Part model, mm, in its own coordinate system. Give positions to 0.01 mm unless a question says otherwise; leave off trailing zeros. Loops run counter-clockwise (first coordinate to the right, second up) from the corner with the lowest first, then second, coordinate; pieces in that order, holes last. Notation, with made-up numbers: M -3,-17 L 12,-17 A8 cw 12,-7 Z; hole C 21,46.5 d2. An arc over 180 degrees is marked long. Put each result on its own line as item: value. Start each with the question number.
Autodesk Inventor part; units mm, degrees
ref_plane "YZ Plane" through (0, 0, 0) normal (1, 0, 0) x (0, 1, 0)
ref_plane "XZ Plane" through (0, 0, 0) normal (0, 1, 0) x (-1, 0, 0)
ref_plane "XY Plane" through (0, 0, 0) normal (0, 0, 1) x (1, 0, 0)
sketch "Boceto3" plane through (0, 0, 0) normal (0, 0, 1) x (1, 0, 0)
  line L0 (25, -3) -> (25, 3)
  line L1 (25, 3) -> (-25, 3)
  line L2 (-25, 3) -> (-25, -3)
  line L3 (-25, -3) -> (25, -3)
  line L4 (25, -3) -> (-25, 3) construction
  line L5 (25, 3) -> (-25, -3) construction
  point P0 (0, 0)
  dimension "d15" = 6
  dimension "d16" = 50
extrude "Extrusión3" add sketch "Boceto3" along normal mid plane 130
sketch "Boceto4" plane through (-25, 3, 65) normal (0, 1, 0) x (1, 0, 0)
  line L0 (40, 102.5) -> (40, 27.5)
  line L1 (40, 27.5) -> (10, 27.5)
  line L2 (10, 27.5) -> (10, 102.5)
  line L3 (10, 102.5) -> (40, 102.5)
  line L4 (40, 102.5) -> (10, 27.5) construction
  line L5 (40, 27.5) -> (10, 102.5) construction
  circle A0 centre (25, 14.5) radius 4
  circle A1 centre (25, 14.5) radius 13
  line L6 (19.6627, 65) -> (30.4742, 65)
  circle A2 centre (25, 115.5) radius 4
  circle A3 centre (25, 115.5) radius 13
  point P0 (25, 65)
  point P1 (25, 65)
  dimension "d19" = 75
  dimension "d20" = 8
  dimension "d21" = 26
extrude "Extrusión4" cut sketch "Boceto4" against normal through all contours A0 | A2
fillet "Empalme2" radius 8 4 edges at (25, 0, 65) (-25, 0, 65) (-25, 0, -65) (25, 0, -65)
properties part number "SIDE BEARING GUIDE" material "Acero"
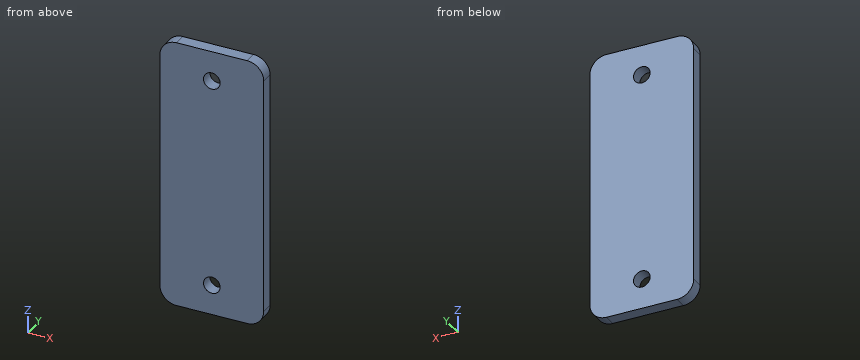
1) Pin check, flat tips, straight feed: pin 1 Ø10.5 at (x, z) = (0, 50.5) entering from +Y; pin 2 Ø5 at (x, z) = (0, -50.5) entering from +Y. Stop position of each tip, or through.
2) Band-saw the part on A-A on x = 0. Give the cut face in (y, z), then the cut area to 3 significant figures.
3) Band-saw the part on B-B on z = 50.5. Give the cut face in (x, y).
4) Wall check: L1, parallel to Z at x = 0, y = 1.85; L2, parallel to X at y = 1.55, z = 50.5; L3, parallel to Z at x = -3, y = 0.3. Give the ranges that are in metal, low to high.
5) Band-saw the part on C-C on y = 0.35. Give the cut face in (x, z).
Evaluation:
1. pin 1: y = 3
1. pin 2: through
2. outline: M -3,-65 L 3,-65 L 3,-54.5 L -3,-54.5 Z; M -3,-46.5 L 3,-46.5 L 3,46.5 L -3,46.5 Z; M -3,54.5 L 3,54.5 L 3,65 L -3,65 Z
2. area: 684 mm2
3. outline: M -25,-3 L -4,-3 L -4,3 L -25,3 Z; M 4,-3 L 25,-3 L 25,3 L 4,3 Z
4. L1: -65 to -54.5, -46.5 to 46.5, 54.5 to 65
4. L2: -25 to -4, 4 to 25
4. L3: -65 to -53.15, -47.85 to 47.85, 53.15 to 65
5. outline: M -25,-57 A8 ccw -17,-65 L 17,-65 A8 ccw 25,-57 L 25,57 A8 ccw 17,65 L -17,65 A8 ccw -25,57 Z; hole C 0,-50.5 d8; hole C 0,50.5 d8
